Check sheet for the modelled part. Datum: model origin and axes. Units: mm. Face numbers are marked on the shaded views. A direction names the side the tool comes from. Round coordinates to 2 decimals unless told otherwise and drop trailing zeros. Write each loop counter-clockwise with the first axis right and the second up, starting at its lowest first coordinate (ties: lowest second). Pieces come first, ordered by that corner, then holes. Notation, with made-up numbers: (7.25, -10.5) -> (63.25, -10.5) arc R34 ccw to (63.25, 27.5) -> close; hole circle Ø11 at (-35, 49.5). An arc over 180 degrees is marked (long way). Write item = value, one per line.
from build123d import *

# Parameters (mm, degrees)
SKETCH1_W           = 8
SKETCH1_H           = 9.5
BOSS_EXTRUDE1_DEPTH = 4.5
SKETCH2_R           = 2
BOSS_EXTRUDE2_DEPTH = 6
CUT_EXTRUDE1_DEPTH  = 1.5
SKETCH6_R           = 2
CUT_EXTRUDE2_DEPTH  = 9
FILLET1_R           = 2


with BuildPart() as part:
    # Sketch1 → Boss-Extrude1 (new body, symmetric)
    with BuildSketch(Plane(origin=(0, 0, 0), x_dir=(1, 0, 0), z_dir=(0, 1, 0))):
        Rectangle(SKETCH1_W, SKETCH1_H)
    extrude(amount=BOSS_EXTRUDE1_DEPTH, both=True)

    # Sketch2 → Boss-Extrude2 (add)
    with BuildSketch(Plane(origin=(0, 4.5, 0), x_dir=(1, 0, 0), z_dir=(0, 1, 0))):
        Circle(SKETCH2_R)
    extrude(amount=BOSS_EXTRUDE2_DEPTH)

    # Sketch5 → Cut-Extrude1 (cut, symmetric)
    with BuildSketch(Plane(origin=(0, 0, 0), x_dir=(0, 0, -1), z_dir=(1, 0, 0))):
        Polygon((-3.5, -2.020725942), (-3.5, -4.5), (3.5, -4.5), (3.5, -2.020725942), (3.5, 2.020725942), (0, 4.041451884), (-3.5, 2.020725942), align=None)
    extrude(amount=CUT_EXTRUDE1_DEPTH, both=True, mode=Mode.SUBTRACT)

    # Sketch6 → Cut-Extrude2 (cut, through all)
    with BuildSketch(Plane(origin=(4, 0, 0), x_dir=(0, 0, -1), z_dir=(1, 0, 0))):
        Circle(SKETCH6_R)
    extrude(amount=-CUT_EXTRUDE2_DEPTH, mode=Mode.SUBTRACT)

    # Fillet1
    fillet1_edges = [part.edges().sort_by_distance(p)[0] for p in [
        (-4, 0, -4.75),
        (4, 0, -4.75),
        (4, 0, 4.75),
        (-4, 0, 4.75),
    ]]
    fillet(fillet1_edges, radius=FILLET1_R)


solid = part.part
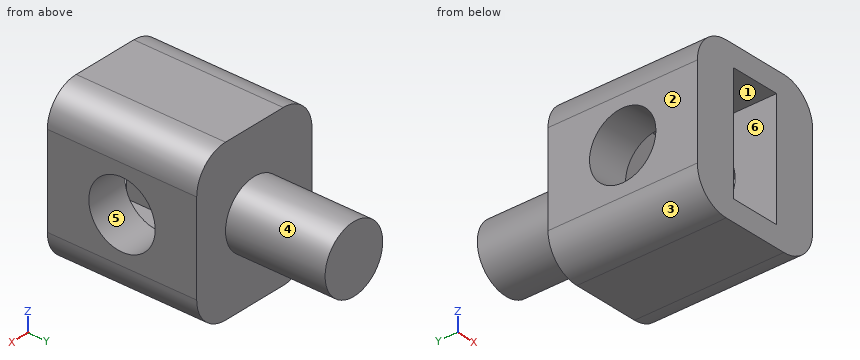
(1) Go/stop test with flat-tipped pins: P1, Ø3, axis at x = 3, z = 0, coming from the +Y side; P2, Ø2.5, axis at y = 0, z = 0, coming from the +X side; P3, Ø1, axis at x = -1.5, z = 3, coming from the +Y side. Record where each tip stops, or that it passes through.
Worked answers:
P1 = 10.5
P2 = through
P3 = 4.5
(2) Material ranges on L1, parallel to Z at x = 0.25, y = -3.25; L2, parallel to Y at x = -2.65, z = 0; L3, parallel to X at y = 3, z = 0.25, recorded low to high. Write a range as [from, to].
Worked answers:
L1 = [-4.75, -3.5], [3.5, 4.75]
L2 = [-4.5, -2], [2, 4.5]
L3 = [-4, -1.5], [1.5, 4]
(3) Sectioned sample at A-A on y = 0. Enter the section's corners in (x, z).
Worked answers:
outline = (-4, -2.75) arc R2 ccw to (-2, -4.75) -> (2, -4.75) arc R2 ccw to (4, -2.75) -> (4, -2) -> (1.5, -2) -> (1.5, -3.5) -> (-1.5, -3.5) -> (-1.5, -2) -> (-4, -2) -> close; (-4, 2) -> (-1.5, 2) -> (-1.5, 3.5) -> (1.5, 3.5) -> (1.5, 2) -> (4, 2) -> (4, 2.75) arc R2 ccw to (2, 4.75) -> (-2, 4.75) arc R2 ccw to (-4, 2.75) -> close
(4) Sectioned sample at D-D on z = -0.75. Enter the section's corners in (x, y).
Worked answers:
outline = (-4, -4.5) -> (-1.5, -4.5) -> (-1.5, -1.85) -> (-4, -1.85) -> close; (-4, 1.85) -> (-1.5, 1.85) -> (-1.5, 3.61) -> (1.5, 3.61) -> (1.5, 1.85) -> (4, 1.85) -> (4, 4.5) -> (1.85, 4.5) -> (1.85, 10.5) -> (-1.85, 10.5) -> (-1.85, 4.5) -> (-4, 4.5) -> close; (1.5, -4.5) -> (4, -4.5) -> (4, -1.85) -> (1.5, -1.85) -> close
(5) Release check for a two-part mould opening along Z. For the marked faces 1, 2, 3 and 4 record: pulls with the +Z half, pulls with the -Z half, needs draft (parallel to the pull), parting line crosses it, or undercut.
Worked answers:
face_1 = undercut
face_2 = needs draft
face_3 = pulls with the -Z half
face_4 = parting line crosses it
(6) Sectioned sample at C-C on y = -3.25. Enter the section's corners in (x, z).
Worked answers:
outline = (-4, -2.75) arc R2 ccw to (-2, -4.75) -> (2, -4.75) arc R2 ccw to (4, -2.75) -> (4, 2.75) arc R2 ccw to (2, 4.75) -> (-2, 4.75) arc R2 ccw to (-4, 2.75) -> close; hole (-1.5, -3.5) -> (1.5, -3.5) -> (1.5, 3.5) -> (-1.5, 3.5) -> close
(7) Access from +Z, -Z, +X, -X, +Y, -Y to the whole of each face (thin tool, end or side, straight path). Record for the marked faces 5 and 6.
Worked answers:
face_5 = +X, -X
face_6 = -Y
(8) Sectioned sample at B-B on x = 0. Enter the section's corners in (y, z).
Worked answers:
outline = (-4.5, -4.75) -> (4.5, -4.75) -> (4.5, -2) -> (10.5, -2) -> (10.5, 2) -> (4.5, 2) -> (4.5, 4.75) -> (-4.5, 4.75) -> (-4.5, 3.5) -> (2.02, 3.5) -> (4.04, 0) -> (2.02, -3.5) -> (-4.5, -3.5) -> close
